Check sheet for the modelled part. Datum: model origin and axes. Units: mm. Face numbers are marked on the shaded views. A direction names the side the tool comes from. Give positions to 0.01 mm unless a question says otherwise; leave off trailing zeros. Loops run counter-clockwise (first coordinate to the right, second up) from the corner with the lowest first, then second, coordinate; pieces in that order, holes last. Notation, with made-up numbers: M 31.5,-34.75 L 37.5,-34.75 A32 ccw 37.5,-5.75 Z; hole C 60.5,15 d8. An arc over 180 degrees is marked long. Use one line per item in the form item = value.
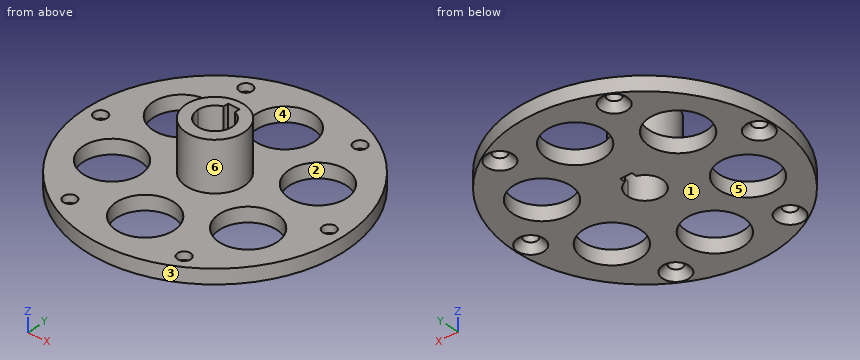
from build123d import *

# Parameters (mm, degrees)
SKETCH1_R                                            = 45
SKETCH1_R_2                                          = 6
EXTRUDE1_DEPTH                                       = 5
SKETCH2_R                                            = 10
SKETCH2_R_2                                          = 6
EXTRUDE2_DEPTH                                       = 22
SKETCH4_R                                            = 10
CUT_EXTRUDE2_DEPTH                                   = 100
SKETCH5_W                                            = 4
SKETCH5_H                                            = 1.8
CUT_EXTRUDE3_DEPTH                                   = 50
SKETCH6_R                                            = 2
CUT_EXTRUDE4_DEPTH                                   = 15
CSK_FOR_M4_HEX_SOCKET_COUNTERSUNK_HEAD_S_D           = 4.5
CSK_FOR_M4_HEX_SOCKET_COUNTERSUNK_HEAD_S_CSINK_D     = 9.18
CSK_FOR_M4_HEX_SOCKET_COUNTERSUNK_HEAD_S_CSINK_ANGLE = 90
CIRPATTERN1_COUNT                                    = 6


with BuildPart() as part:
    # Sketch1 → Extrude1 (new body)
    with BuildSketch(Plane.XY):
        Circle(SKETCH1_R)
        Circle(SKETCH1_R_2, mode=Mode.SUBTRACT)
    extrude(amount=EXTRUDE1_DEPTH)

    # Sketch2 → Extrude2 (add)
    with BuildSketch(Plane(origin=(0, 0, 0), x_dir=(-1, 0, 0), z_dir=(0, 0, -1))):
        Circle(SKETCH2_R)
        Circle(SKETCH2_R_2, mode=Mode.SUBTRACT)
    extrude(amount=-EXTRUDE2_DEPTH)

    # Sketch4 → Cut-Extrude2 (cut)
    with BuildSketch(Plane.XY.offset(5)):
        with Locations((23.815698604, 13.75)):
            Circle(SKETCH4_R)
        with Locations((0, 27.5)):
            Circle(SKETCH4_R)
        with Locations((23.815698604, -13.75)):
            Circle(SKETCH4_R)
        with Locations((0, -27.5)):
            Circle(SKETCH4_R)
        with Locations((-23.815698604, -13.75)):
            Circle(SKETCH4_R)
        with Locations((-23.815698604, 13.75)):
            Circle(SKETCH4_R)
    extrude(amount=-CUT_EXTRUDE2_DEPTH, mode=Mode.SUBTRACT)

    # Sketch5 → Cut-Extrude3 (cut)
    with BuildSketch(Plane.XY.offset(22)):
        with Locations((0, 6.556854249)):
            Rectangle(SKETCH5_W, SKETCH5_H)
    extrude(amount=-CUT_EXTRUDE3_DEPTH, mode=Mode.SUBTRACT)

    # Sketch6 → Cut-Extrude4 (cut)
    with BuildSketch(Plane(origin=(0, 0, 0), x_dir=(-1, 0, 0), z_dir=(0, 0, -1))):
        with Locations((20, 34.641016151)):
            Circle(SKETCH6_R)
    extrude(amount=-CUT_EXTRUDE4_DEPTH, mode=Mode.SUBTRACT)

    # CSK for M4 Hex Socket Countersunk Head S (through all)
    with Locations(Plane(origin=(-20, 34.641016151, 0), x_dir=(-1, 0, 0), z_dir=(0, 0, -1))):
        with Locations((0, 0)):
            csk_for_m4_hex_socket_countersunk_head_s = CounterSinkHole(CSK_FOR_M4_HEX_SOCKET_COUNTERSUNK_HEAD_S_D / 2, CSK_FOR_M4_HEX_SOCKET_COUNTERSUNK_HEAD_S_CSINK_D / 2, counter_sink_angle=CSK_FOR_M4_HEX_SOCKET_COUNTERSUNK_HEAD_S_CSINK_ANGLE)

    # CirPattern1: CSK for M4 Hex Socket Countersunk Head S ×6 about axis
    cirpattern1_axis = Axis((0, 0, 0), (0, 0, 1))
    for i in range(1, CIRPATTERN1_COUNT):
        add(csk_for_m4_hex_socket_countersunk_head_s.rotate(cirpattern1_axis, i * 360 / CIRPATTERN1_COUNT), mode=Mode.SUBTRACT)


solid = part.part
1) Section check D-D (y = -27.5). Record the cut outline in (x, z), then the cut area to 3 significant figures.
Evaluation:
outline = M -35.62,0 L -10,0 L -10,5 L -35.62,5 Z; M 10,0 L 35.62,0 L 35.62,5 L 10,5 Z
area = 256 mm^2
2) Scan lines: line 1 (Y direction, x = 0, z = 3.1); line 2 (Y direction, x = 20, z = 3.5); line 3 (Z direction, x = -22, y = 1). Record each from-to range of solid material in increasing order.
Evaluation:
line_1 = -45 to -37.5, -17.5 to -6, 7.46 to 17.5, 37.5 to 45
line_2 = -40.31 to -36.89, -32.39 to -22.99, -4.51 to 4.51, 22.99 to 32.39, 36.89 to 40.31
line_3 = 0 to 5
3) Release check for a two-part mould opening along Y. For the marked faces 1, 2, 3 and 4 record: pulls with the +Y half, pulls with the -Y half, needs draft (parallel to the pull), parting line crosses it, or undercut.
Evaluation:
face_1 = needs draft
face_2 = undercut
face_3 = parting line crosses it
face_4 = undercut
4) Section check B-B (z = 15.75). Record the cut outline in (x, y), then the cut area to 3 significant figures.
Evaluation:
outline = C 0,0 d20; hole M -2,5.66 A6 ccw long 2,5.66 L 2,7.46 L -2,7.46 Z
area = 195 mm^2
5) Section check A-A (x = 0). Record the cut outline in (y, z).
Evaluation:
outline = M -45,0 L -37.5,0 L -37.5,5 L -45,5 Z; M -17.5,0 L -6,0 L -6,22 L -10,22 L -10,5 L -17.5,5 Z; M 7.46,0 L 17.5,0 L 17.5,5 L 10,5 L 10,22 L 7.46,22 Z; M 37.5,0 L 45,0 L 45,5 L 37.5,5 Z
6) Depth check by flat-ended pin: pin 1 Ø1.5 at (x, y) = (-11.5, -12) entering from +Z; pin 2 Ø6 at (x, y) = (-40, 0) entering from -Z; pin 3 Ø8 at (y, z) = (30, 5) entering from +X; pin 4 Ø10 at (x, y) = (3.5, -10) entering from -Z. Enter the tip coordinate at first touch or a pass-through.
Evaluation:
pin_1 = 5
pin_2 = 1.59
pin_3 = 36.73
pin_4 = 0
7) Set-up check for the marked faces 5 and 6: record each of +Z, -Z, +X, -X, +Y, -Y from which the full face is reachable in a straight line by a thin tool's end or side.
Evaluation:
face_5 = +Z, -Z
face_6 = +Z
8) Section check C-C (x = -40). Record the cut outline in (y, z).
Evaluation:
outline = M -20.62,0 L -4.59,0 L -2.25,2.34 L -2.25,5 L -20.62,5 Z; M 2.25,2.34 L 4.59,0 L 20.62,0 L 20.62,5 L 2.25,5 Z
